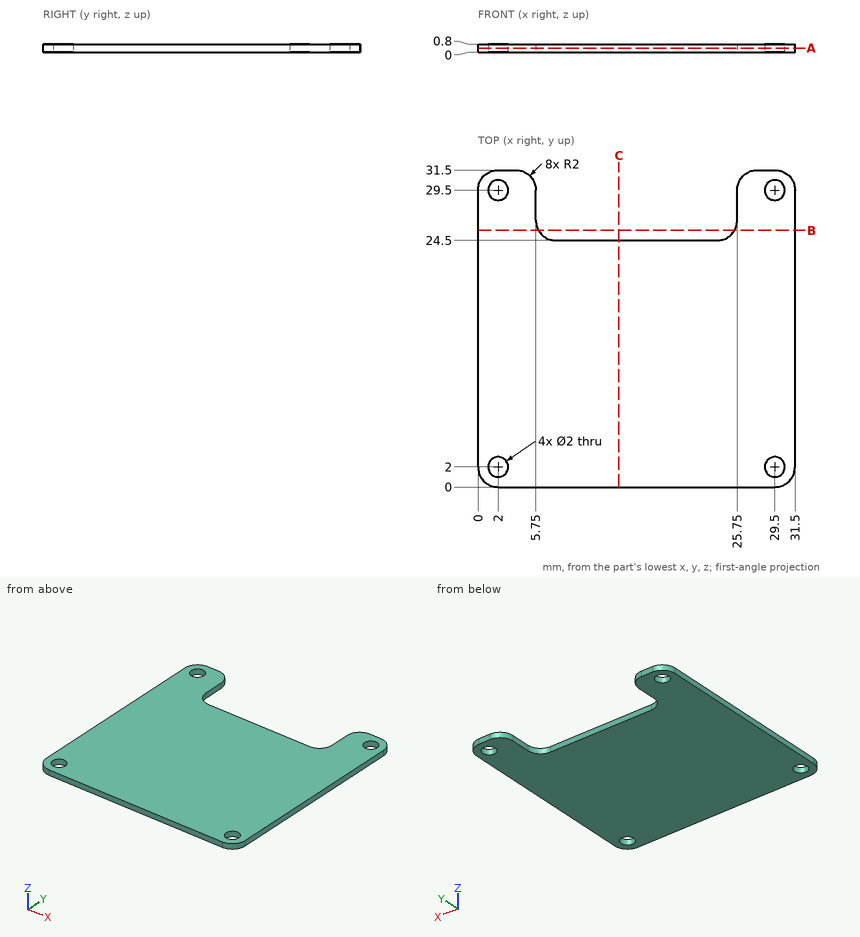
Study the drawing (mm; zero at the part's minimum x, y, z) and answer. Coordinates: 2 decimals unless noted, no trailing zeros. Loops run counter-clockwise (first coordinate to the right, second up) from the corner with the lowest first, then second, coordinate; pieces in that order, holes last. Notation, with made-up numbers: M 65.5,-24 L 96.5,-24 A22 cw 96.5,11 Z; hole C -25,-0.5 d7. An arc over 180 degrees is marked long. Answer in a Markdown table with one row per item. Add a question column.
1. Find section A-A, the plane z = 0.4. Write down the section's boundary in (x, y).
2. Consider L1, parallel to Y at x = 29.5, z = 0.3; L2, parallel to Y at x = 16.5, z = 0.2; L3, parallel to Y at x = 1.5, z = 0.65. Determine where each line is inside the solid, lowest interval first.
3. Find section B-B, the plane y = 25.5. Write down the section's boundary in (x, z), then the cut area to 3 significant figures.
4. Find section C-C, the plane x = 14. Write down the section's boundary in (y, z), then the cut area to 3 significant figures.
Reported:
| question | item | result |
|---|---|---|
| 1 | outline | M 0,2 A2 ccw 2,0 L 29.5,0 A2 ccw 31.5,2 L 31.5,29.5 A2 ccw 29.5,31.5 L 27.75,31.5 A2 ccw 25.75,29.5 L 25.75,26.5 A2 cw 23.75,24.5 L 7.75,24.5 A2 cw 5.75,26.5 L 5.75,29.5 A2 ccw 3.75,31.5 L 2,31.5 A2 ccw 0,29.5 Z; hole C 2,2 d2; hole C 2,29.5 d2; hole C 29.5,2 d2; hole C 29.5,29.5 d2 |
| 2 | L1 | y = 0 to 1, 3 to 28.5, 30.5 to 31.5 |
| 2 | L2 | y = 0 to 24.5 |
| 2 | L3 | y = 0.06 to 1.13, 2.87 to 28.63, 30.37 to 31.44 |
| 3 | outline | M 0,0 L 6.02,0 L 6.02,0.8 L 0,0.8 Z; M 25.48,0 L 31.5,0 L 31.5,0.8 L 25.48,0.8 Z |
| 3 | area | 9.63 mm^2 |
| 4 | outline | M 0,0 L 24.5,0 L 24.5,0.8 L 0,0.8 Z |
| 4 | area | 19.6 mm^2 |
